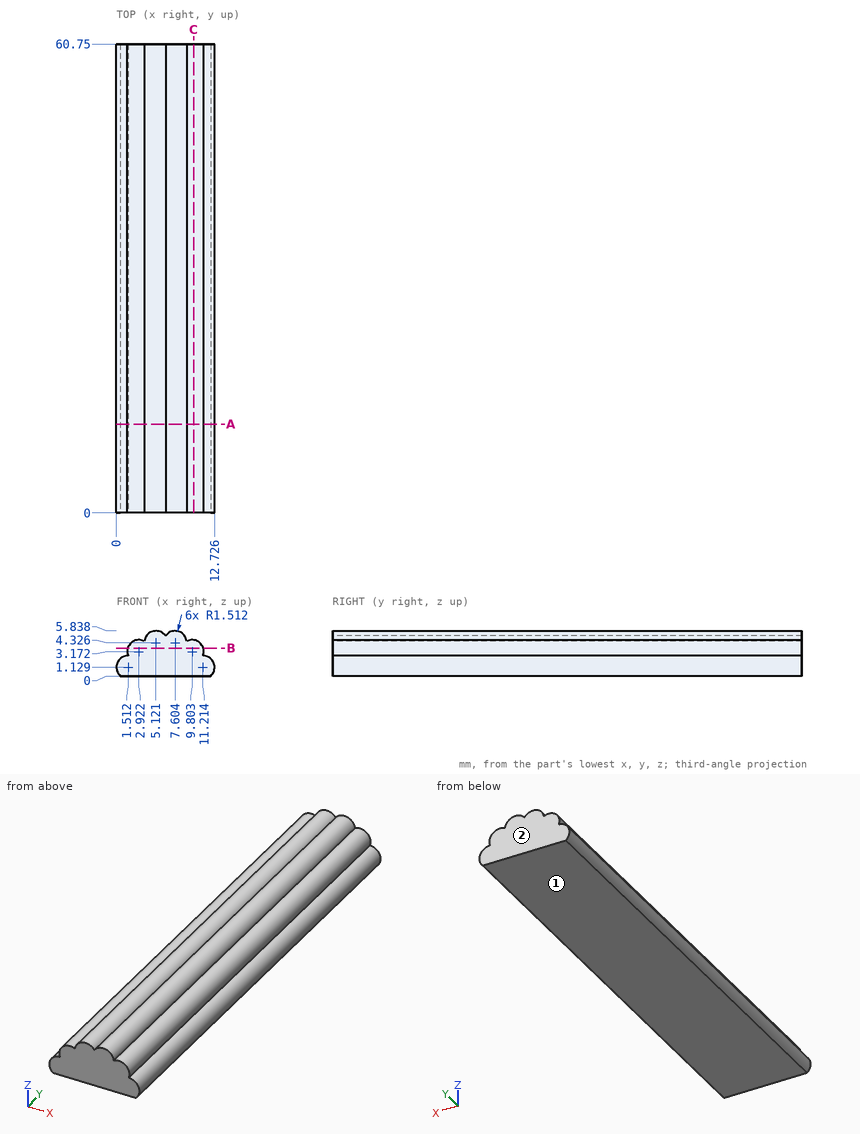
Geometry check sheet. Reference: drawing and pictorial views, mm from the part's lowest x, y, z. Coordinates: 2 decimals unless noted, no trailing zeros. Loops run counter-clockwise (first coordinate to the right, second up) from the corner with the lowest first, then second, coordinate; pieces in that order, holes last.
1) Sectioned sample at B-B (z = 3.6). Record the boundary of the cut face in (x, y), and give its area (3 significant figures).
2) Gauge pin test, flat end, axial feed: pin 1 (2 mm diameter, centred on y = 12.5, z = 5, fed in from -X). Record the tip position at first contact, or that the pin passes through.
3) Material ranges on probe 1 along Z at (x, y) = (2.25, 49) (1 decimal); probe 2 along Z at (x, y) = (7.5, 7) (1 decimal); probe 3 along X at (y, z) = (53.5, 3.5), recorded low to high.
4) Sectioned sample at A-A (y = 11.5). Record the boundary of the cut face in (x, z) (1 decimal), and give its area (3 significant figures).
5) Release check for a two-part mould opening along Z. For the marked faces 1 and 2 record: released by +Z, released by -Z, zero draft, split by the parting line, or undercut.
6) Sectioned sample at C-C (x = 10). Record the boundary of the cut face in (y, z).
Check sheet entries:
1. outline: (1.47, 0) - (11.25, 0) - (11.25, 60.75) - (1.47, 60.75) - close
1. area: 594 mm2
2. pin 1: stops at x = 1.66
3. probe 1: z = 0 to 4.5
3. probe 2: z = 0 to 5.8
3. probe 3: x = 1.45 to 11.28
4. outline: (0.5, 0) - (12.2, 0) arc R1.5 ccw to (11.2, 2.6) arc R1.5 ccw to (9.1, 4.5) arc R1.5 ccw to (6.4, 5.2) arc R1.5 ccw to (3.6, 4.5) arc R1.5 ccw to (1.5, 2.6) arc R1.5 ccw to start
4. area: 56.3 mm2
5. face 1: released by -Z
5. face 2: zero draft
6. outline: (0, 0) - (60.75, 0) - (60.75, 4.67) - (0, 4.67) - close
